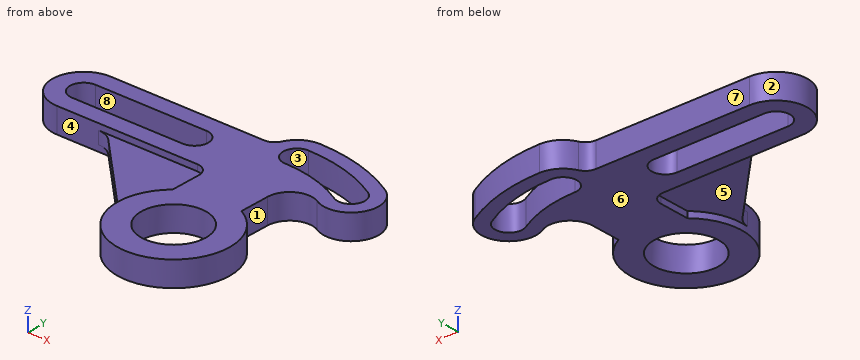
```python
from build123d import *

# Parameters (mm, degrees)
SKETCH_1_R      = 26
EXTRUDE_1_DEPTH = 10
EXTRUDE_2_DEPTH = 5
FILLET_1_R      = 18


with BuildPart() as part:
    # Sketch 1 → Extrude 1 (new, symmetric)
    with BuildSketch(Plane.XY):
        with BuildLine():
            ThreePointArc((46.5, -12.459637448), (28.753378996, -12.882823889), (20, -28.326269101))
            Line((20, -28.326269101), (20, -52.688711259))
            ThreePointArc((20, -52.688711259), (6.038140099, -137.593058475), (-30, -59.458980338))
            Line((-30, -59.458980338), (-30, -35))
            ThreePointArc((-30, -35), (-32.928932188, -27.928932188), (-40, -25))
            Line((-40, -25), (-154, -25))
            ThreePointArc((-154, -25), (-179, 0), (-154, 25))
            Line((-154, 25), (-29.240383034, 25))
            ThreePointArc((-29.240383034, 25), (-23.791759355, 26.614745084), (-20.102763336, 30.9375))
            ThreePointArc((-20.102763336, 30.9375), (-11.986972095, 40.447560814), (0, 44))
            ThreePointArc((0, 44), (35.458209179, 39.331838202), (68.5, 25.645480318))
            ThreePointArc((68.5, 25.645480318), (76.552558883, -4.407078565), (46.5, -12.459637448))
        make_face()
        with Locations((0, -93)):
            Circle(SKETCH_1_R, mode=Mode.SUBTRACT)
        with BuildLine():
            ThreePointArc((0, 33), (-11, 22), (0, 11))
            ThreePointArc((0, 11), (26.917180691, 7.456285934), (52, -2.933358006))
            ThreePointArc((52, -2.933358006), (67.026279442, 1.092921435), (63, 16.119200877))
            ThreePointArc((63, 16.119200877), (32.611199683, 28.706654112), (0, 33))
        make_face(mode=Mode.SUBTRACT)
        with BuildLine():
            ThreePointArc((-64, -11), (-53, 0), (-64, 11))
            Line((-64, 11), (-154, 11))
            ThreePointArc((-154, 11), (-165, 0), (-154, -11))
            Line((-154, -11), (-64, -11))
        make_face(mode=Mode.SUBTRACT)
    extrude(amount=EXTRUDE_1_DEPTH, both=True)

    # Sketch 1_3 → Extrude 2 (add, symmetric)
    with BuildSketch(Plane.XY):
        with BuildLine():
            Line((-30, -59.458980338), (-30, -35))
            ThreePointArc((-30, -35), (-32.928932188, -27.928932188), (-40, -25))
            Line((-40, -25), (-113, -25))
            Line((-113, -25), (-45, -93))
            ThreePointArc((-45, -93), (-41.079191813, -74.628826929), (-30, -59.458980338))
        make_face()
    extrude(amount=EXTRUDE_2_DEPTH, both=True)

    # Fillet 1
    fillet_1_edges = [part.edges().sort_by_distance(p)[0] for p in [
        (-113, -25, 0),
        (-45, -93, 0),
    ]]
    fillet(fillet_1_edges, radius=FILLET_1_R)


solid = part.part
```
Geometry check sheet. Reference: the model listing, model coordinates, mm. Face numbers are marked on the shaded views. A direction names the side the tool comes from. Give positions to 0.01 mm unless a question says otherwise; leave off trailing zeros. Write each loop counter-clockwise with the first axis right and the second up, starting at its lowest first coordinate (ties: lowest second). Pieces come first, ordered by that corner, then holes.
1) Section check C-C, the plane y = -48. Record the boundary of the cut face in (x, z), and give its area (3 significant figures).
2) Gauge pin test, flat ends, axial feed: pin 1 (1.5 mm diameter, centred on y = -91.5, z = -3, fed in from -X); pin 2 (22 mm diameter, centred on x = -62, y = -80, fed in from +Z); pin 3 (10 mm diameter, centred on x = -106, z = -5, fed in from +Y). Record the tip position at first contact, or that the pin passes through.
3) Section check A-A, the plane x = -92. Record the boundary of the cut face in (y, z), and give its area (3 significant figures).
4) Access from +Z, -Z, +X, -X, +Y, -Y to the whole of each face (thin tool, end or side, straight path). Record for the marked faces 5, 6, 7 and 8.
5) Release check for a two-part mould opening along X. For the marked faces 1, 2, 3 and 4 record: pulls with the +X half, pulls with the -X half, needs draft (parallel to the pull), parting line crosses it, or undercut.
6) Material ranges on L1, parallel to Y at x = -144, z = 5.75; L2, parallel to X at y = 2, z = -4; L3, parallel to X at y = -40.5, z = -7, recorded low to high.
7) Section check D-D, the plane z = -0.5. Record the boundary of the cut face in (x, y) (1 decimal).
8) Section check B-B, the plane y = -93. Record the boundary of the cut face in (x, z).
Computed:
1. outline: (-90, -5) - (-30, -5) - (-30, -10) - (20, -10) - (20, 10) - (-30, 10) - (-30, 5) - (-90, 5) - close
1. area: 1,600 mm2
2. pin 1: stops at x = -47.67
2. pin 2: stops at z = 5
2. pin 3: stops at y = 25
3. outline: (-46, -5) - (-25, -5) - (-25, -10) - (-11, -10) - (-11, 10) - (-25, 10) - (-25, 5) - (-46, 5) - close; (11, -10) - (25, -10) - (25, 10) - (11, 10) - close
3. area: 770 mm2
4. face 5: -Z, -X
4. face 6: -Z, +X, -X, +Y, -Y
4. face 7: +Z, -Z, -X, +Y
4. face 8: +Z, -Z
5. face 1: pulls with the +X half
5. face 2: pulls with the -X half
5. face 3: undercut
5. face 4: needs draft
6. L1: y = -25 to -11, 11 to 25
6. L2: x = -178.92 to -164.82, -53.18 to 42.32, 67.5 to 79.02
6. L3: x = -30 to 20
7. outline: (-154, -25) - (-120.5, -25) arc R18 cw to (-107.7, -30.3) - (-49.8, -88.2) arc R18 cw to (-44.6, -98.7) arc R45 ccw (long way) to (20, -52.7) - (20, -28.3) arc R18 cw to (46.5, -12.5) arc R22 ccw to (68.5, 25.6) arc R137 ccw to (0, 44) arc R22 ccw to (-20.1, 30.9) arc R10 cw to (-29.2, 25) - (-154, 25) arc R25 ccw to start; hole (-154, -11) - (-64, -11) arc R11 ccw to (-64, 11) - (-154, 11) arc R11 ccw to start; hole circle Ø52 at (0, -93); hole (0, 11) arc R104 cw to (52, -2.9) arc R11 ccw to (63, 16.1) arc R126 ccw to (0, 33) arc R11 ccw to start
8. outline: (-46.35, -5) - (-45, -5) - (-45, -10) - (-26, -10) - (-26, 10) - (-45, 10) - (-45, 5) - (-46.35, 5) - close; (26, -10) - (45, -10) - (45, 10) - (26, 10) - close
